Model file for the job. Use its own axes, mm. A direction names the side the tool comes from. Coordinates: 2 decimals unless noted, no trailing zeros. Order: outer loops, then holes, each group sorted by start corner. A loop starts at its lowest first (then second) coordinate and runs counter-clockwise, first axis right, second up.
from build123d import *

# Parameters (mm, degrees)
SKETCH1_W           = 30
SKETCH1_H           = 6
BOSS_EXTRUDE1_DEPTH = 7.9
SKETCH2_R           = 1.5
CUT_EXTRUDE1_DEPTH  = 32.597626493


with BuildPart() as part:
    # Sketch1 → Boss-Extrude1 (new body)
    with BuildSketch(Plane.XY):
        with Locations((15, 3)):
            Rectangle(SKETCH1_W, SKETCH1_H)
        with BuildLine():
            ThreePointArc((13.581884058, 3.843473281), (9.35, 3), (13.581884058, 2.156526719))
            ThreePointArc((13.581884058, 2.156526719), (15, 1.35), (16.418115942, 2.156526719))
            ThreePointArc((16.418115942, 2.156526719), (20.65, 3), (16.418115942, 3.843473281))
            ThreePointArc((16.418115942, 3.843473281), (15, 4.65), (13.581884058, 3.843473281))
        make_face(mode=Mode.SUBTRACT)
    extrude(amount=BOSS_EXTRUDE1_DEPTH)

    # Sketch2 → Cut-Extrude1 (cut, through all)
    with BuildSketch(Plane(origin=(0, 6, 0), x_dir=(1, 0, 0), z_dir=(0, 1, 0))):
        with Locations(Location((3, -3.95, 0), (0, 0, 270))):
            Circle(SKETCH2_R)
        with Locations(Location((27, -3.95, 0), (0, 0, 270))):
            Circle(SKETCH2_R)
    extrude(amount=-CUT_EXTRUDE1_DEPTH, mode=Mode.SUBTRACT)


solid = part.part
Q1. Cut at B-B, the plane z = 3.95. List the corners of the cut face in (x, y).
Established:
outline: (0, 0) - (1.5, 0) - (1.5, 6) - (0, 6) - close; (4.5, 0) - (25.5, 0) - (25.5, 6) - (4.5, 6) - close; (28.5, 0) - (30, 0) - (30, 6) - (28.5, 6) - close; hole (13.58, 2.16) arc R1.65 ccw to (16.42, 2.16) arc R2.2 ccw (long way) to (16.42, 3.84) arc R1.65 ccw to (13.58, 3.84) arc R2.2 ccw (long way) to start
Q2. Cut at C-C, the plane y = 3. List the corners of the cut face in (x, z).
Established:
outline: (0, 0) - (9.35, 0) - (9.35, 7.9) - (0, 7.9) - close; (20.65, 0) - (30, 0) - (30, 7.9) - (20.65, 7.9) - close; hole circle Ø3 at (3, 3.95); hole circle Ø3 at (27, 3.95)
Q3. Mould opens along X. For faces 3 (the face through (14.98, 1.35, 3.89)), 4 (the face through (15, 5, 0)), 5 (the face through (0, 3, 4)), 6 (the face through (1.536, 3.042, 3.625)) say: pulls with the +X half, pulls with the -X half, needs draft (parallel to the pull), parting line crosses it, or undercut.
Established:
face 3: undercut
face 4: needs draft
face 5: pulls with the -X half
face 6: undercut
Q4. Which spindle directions (+Z, -Z, +X, -X, +Y, -Y) get a long thin tool onto all of the face, cutting with end or side? Do faces 1 (the face through (15, 5, 7.9)), 2 (the face through (15.02, 4.65, 3.89)). Say none if no direction does.
Established:
face 1: +Z, +X, -X, +Y, -Y
face 2: +Z, -Z
Q5. Probe line 1 (X direction, y = 5.4, z = 4.75); line 2 (Y direction, x = 11.55, z = 2); line 3 (X direction, y = 4.25, z = 3.95). List the from-to ranges inside material, lowest first.
Established:
line 1: x = 0 to 1.73, 4.27 to 25.73, 28.27 to 30
line 2: y = 0 to 0.8, 5.2 to 6
line 3: x = 0 to 1.5, 4.5 to 9.74, 13.36 to 13.92, 16.08 to 16.64, 20.26 to 25.5, 28.5 to 30
Q6. Cut at A-A, the plane x = 11.55. List the corners of the cut face in (y, z), plus the area to 3 significant figures.
Established:
outline: (0, 0) - (0.8, 0) - (0.8, 7.9) - (0, 7.9) - close; (5.2, 0) - (6, 0) - (6, 7.9) - (5.2, 7.9) - close
area: 12.6 mm2
Q7. Drop a flat-ended pin along its axis: P1, Ø2.5, axis at x = 11.55, y = 3, coming from the +Z side. Give the stop position or say it passes through.
Established:
P1: passes through
Q8. Cut at D-D, the plane y = 1.7. List the corners of the cut face in (x, z).
Established:
outline: (0, 0) - (9.78, 0) - (9.78, 7.9) - (0, 7.9) - close; (13.32, 0) - (13.98, 0) - (13.98, 7.9) - (13.32, 7.9) - close; (16.02, 0) - (16.68, 0) - (16.68, 7.9) - (16.02, 7.9) - close; (20.22, 0) - (30, 0) - (30, 7.9) - (20.22, 7.9) - close; hole circle Ø3 at (3, 3.95); hole circle Ø3 at (27, 3.95)
